Source: CAD feature listing. Evaluate the final solid. Frame: model axes, mm. Face numbers are marked on the shaded views. A direction names the side the tool comes from. Round coordinates to 2 decimals unless told otherwise and drop trailing zeros. Write each loop counter-clockwise with the first axis right and the second up, starting at its lowest first coordinate (ties: lowest second). Pieces come first, ordered by that corner, then holes. Notation, with made-up numbers: (-18, -33) -> (39, -33) arc R25 cw to (39, -17) -> close; hole circle Ø11 at (25, 41). An arc over 180 degrees is marked (long way). Put each result on its own line as item: value.
```python
from build123d import *

# Parameters (mm, degrees)
F0_R     = 15
F1_DEPTH = 111.9
F3_W     = 12
F3_H     = 20
F4_DEPTH = 137.6


with BuildPart() as f1:
    # F0 (on Top) → F1 (new body)
    with BuildSketch(Plane.XY):
        Circle(F0_R)
    extrude(amount=F1_DEPTH)

    # F3 (on face) → F4 (join)
    with BuildSketch(Plane(origin=(0, 0, 0), x_dir=(1, 0, 0), z_dir=(0, -0.7071067812, -0.7071067812))):
        with Locations((0, 10)):
            Rectangle(F3_W, F3_H)
    extrude(amount=-F4_DEPTH)


solid = f1.part
```
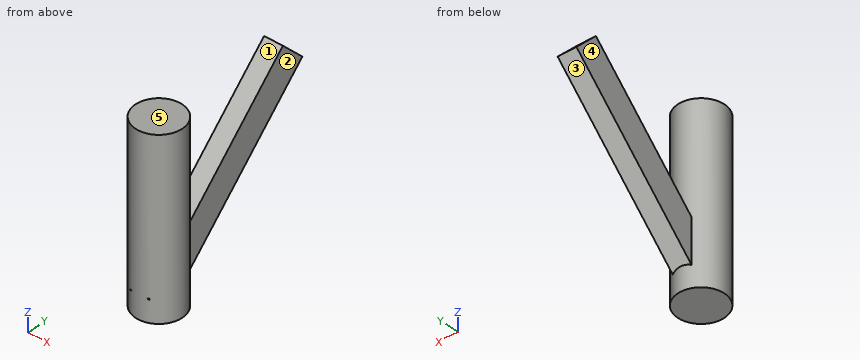
Q1. Cut plane C-C on y = 33.5. Output: boundary loops of the cut face in (x, z).
Ans:
outline: (-6, 33.5) -> (6, 33.5) -> (6, 61.78) -> (-6, 61.78) -> close
Q2. Draft query along Y for the marked faces 1, 2 and 3. Return one class per face: +Y half, -Y half, draft (parallel to the pull), parting line (faces both ways), or undercut.
Ans:
face 1: undercut
face 2: draft
face 3: +Y half
Q3. Pin query (flat end, axial travel): pin 1 (25 mm diameter, centred on y = 39, z = 49, fed in from +X); pin 2 (12 mm diameter, centred on x = 6, y = 51.5, fed in from +Z); pin 3 (5 mm diameter, centred on x = 7, z = 77, fed in from -Y). Return the tip coordinate at first contact, or that it passes through.
Ans:
pin 1: stops at x = 6
pin 2: stops at z = 85.78
pin 3: stops at y = -14.31
Q4. Cut plane B-B on x = 0. Output: boundary loops of the cut face in (y, z), and give its area (3 significant figures).
Ans:
outline: (-15, 0) -> (15, 0) -> (15, 15) -> (97.3, 97.3) -> (83.16, 111.44) -> (15, 43.28) -> (15, 111.9) -> (-15, 111.9) -> close
area: 5,480 mm^2
Q5. Reachability of the marked faces 4 and 5 from +Z, -Z, +X, -X, +Y, -Y: full face, straight path, thin tool, end or side. Return the list, or none.
Ans:
face 4: +Z, -Z, -X, +Y
face 5: +Z, +X, -X, +Y, -Y
Q6. Cut plane A-A on z = 58.5. Output: boundary loops of the cut face in (x, y), and give its area (3 significant figures).
Ans:
outline: circle Ø30 at (0, 0); (-6, 30.22) -> (6, 30.22) -> (6, 58.5) -> (-6, 58.5) -> close
area: 1,050 mm^2
Q7. Material intervals for line 1 (X direction, y = 17, z = 27.5); line 2 (Y direction, x = 1.75, z = 43.5); line 3 (Y direction, x = -0.5, z = 50), sorted ascending. Write a range as [from, to].
Ans:
line 1: x = [-6, 6]
line 2: y = [-14.9, 14.9], [15.22, 43.5]
line 3: y = [-14.99, 14.99], [21.72, 50]
Q8. Cut plane D-D on x = -12.25. Output: boundary loops of the cut face in (y, z), and give its area (3 significant figures).
Ans:
outline: (-8.66, 0) -> (8.66, 0) -> (8.66, 111.9) -> (-8.66, 111.9) -> close
area: 1,940 mm^2
